Input: dimensioned drawing with shaded views. Units: mm. Origin: part minimum x, y, z. A direction names the side the tool comes from. Coordinates: 2 decimals unless noted, no trailing zeros. Loops run counter-clockwise (first coordinate to the right, second up) from the corner with the lowest first, then second, coordinate; pieces in that order, holes last.
(1) Set-up query: the marked faces 1 and 2. Return all of +Z, -Z, +X, -X, +Y, -Y with unobstructed straight access to the full face (end or side cutting, diameter ignored); none if empty.
(2) Section C-C, the plane y = 3.55. Return loops of the section in (x, z), then the cut area to 3 significant figures.
(3) Section A-A, the plane z = 3.5. Return loops of the section in (x, y), then the cut area to 3 significant figures.
(4) Section B-B, the plane y = 1.3. Return loops of the section in (x, z), then the cut area to 3 significant figures.
(5) Line query: L1, parallel to Z at x = 3.5, y = 3.05; L2, parallel to Z at x = 3.5, y = 2.35; L3, parallel to X at y = 2.6, z = 4. Output: solid intervals per line, ascending.
(6) Mould query, pull axis Z, two halves, no side actions, for the marked faces 3 and 4. Classes: released by +Z, released by -Z, zero draft, split by the parting line, or undercut.
(7) Contact query for a flat-ended pin moving along its axis: P1, Ø1.5, axis at y = 3, z = 4.5, coming from the -X side. Output: stop coordinate, or through.
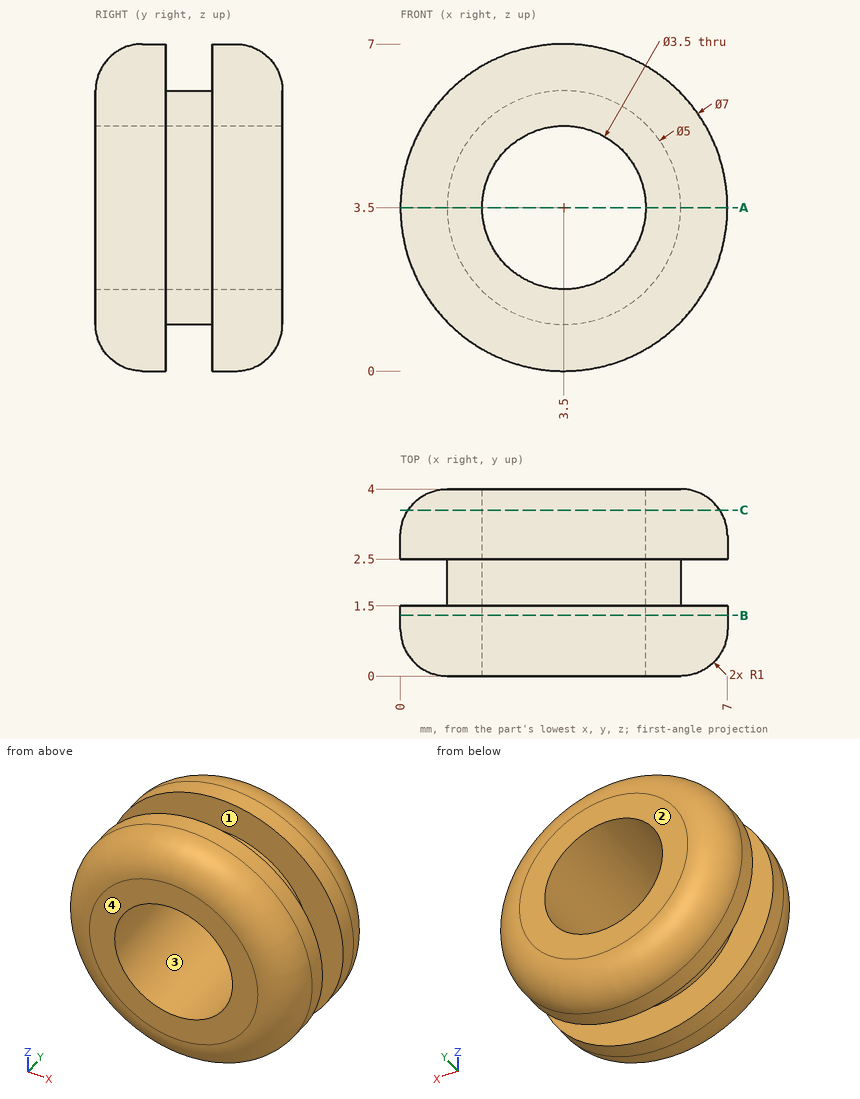
Report:
1. face 1: none
1. face 2: +Z, -Z, +X, -X, +Y
2. outline: circle Ø6.67 at (3.5, 3.5); hole circle Ø3.5 at (3.5, 3.5)
2. area: 25.3 mm2
3. outline: (0, 1) arc R1 ccw to (1, 0) - (1.75, 0) - (1.75, 4) - (1, 4) arc R1 ccw to (0, 3) - (0, 2.5) - (1, 2.5) - (1, 1.5) - (0, 1.5) - close; (5.25, 0) - (6, 0) arc R1 ccw to (7, 1) - (7, 1.5) - (6, 1.5) - (6, 2.5) - (7, 2.5) - (7, 3) arc R1 ccw to (6, 4) - (5.25, 4) - close
3. area: 11.1 mm2
4. outline: circle Ø7 at (3.5, 3.5); hole circle Ø3.5 at (3.5, 3.5)
4. area: 28.9 mm2
5. L1: z = 0 to 1.75, 5.25 to 7
5. L2: z = 1 to 1.75, 5.25 to 6
5. L3: x = 0.04 to 1.82, 5.18 to 6.96
6. face 3: undercut
6. face 4: zero draft
7. P1: stops at x = 0.01
